```python
from build123d import *

# Parameters (mm, degrees)
SKETCH1_R           = 45
SKETCH1_R_2         = 1.2573
BOSS_EXTRUDE2_DEPTH = 2.5
BOSS_EXTRUDE4_START = -2.5
BOSS_EXTRUDE4_DEPTH = 2.5
CIRPATTERN1_COUNT   = 6
CUT_EXTRUDE2_DEPTH  = 2.5
SKETCH6_R           = 1.5
CUT_EXTRUDE3_DEPTH  = 5


with BuildPart() as part:
    # Sketch1 → Boss-Extrude2 (new body)
    with BuildSketch(Plane(origin=(0, 0, 0), x_dir=(1, 0, 0), z_dir=(0, 1, 0))):
        with Locations(Location((0, 0, 0), (0, 0, 270))):
            Circle(SKETCH1_R)
        with Locations(Location((-4.955, -33.87, 0), (0, 0, 270))):
            Circle(SKETCH1_R_2, mode=Mode.SUBTRACT)
        with Locations(Location((4.955, -33.87, 0), (0, 0, 90))):
            Circle(SKETCH1_R_2, mode=Mode.SUBTRACT)
        with Locations(Location((-4.955, 13.84, 0), (0, 0, 270))):
            Circle(SKETCH1_R_2, mode=Mode.SUBTRACT)
        with Locations(Location((4.955, 13.84, 0), (0, 0, 90))):
            Circle(SKETCH1_R_2, mode=Mode.SUBTRACT)
        Polygon((-9.9, -25), (-9.9, 0), (-9.9, 10), (9.9, 10), (9.9, 0), (9.9, -25), align=None, mode=Mode.SUBTRACT)
        with BuildLine():
            Line((-22.25, 22), (-22.25, -22))
            ThreePointArc((-22.25, -22), (-19.25, -25), (-16.25, -22))
            Line((-16.25, -22), (-16.25, 22))
            ThreePointArc((-16.25, 22), (-19.25, 25), (-22.25, 22))
        make_face(mode=Mode.SUBTRACT)
        with BuildLine():
            Line((16.25, 22), (16.25, -22))
            ThreePointArc((16.25, -22), (19.25, -25), (22.25, -22))
            Line((22.25, -22), (22.25, 22))
            ThreePointArc((22.25, 22), (19.25, 25), (16.25, 22))
        make_face(mode=Mode.SUBTRACT)
    extrude(amount=BOSS_EXTRUDE2_DEPTH)

    # Sketch2 → Boss-Extrude4 (add)
    with BuildSketch(Plane(origin=(0, 2.5, 0), x_dir=(1, 0, 0), z_dir=(0, 1, 0)).offset(BOSS_EXTRUDE4_START)):
        with BuildLine():
            ThreePointArc((-42.23454554, 15.532004475), (-45, 0), (-42.23454554, -15.532004475))
            add(Edge.make_bspline(
                [(-50.212380227, -7.942360629), (-45.3159648, -11.95963121), (-42.656686571, -14.489512492), (-42.23454554, -15.532004475)],
                knots=[0.089311832, 0.089311832, 0.089311832, 0.089311832, 1, 1, 1, 1], degree=3))
            ThreePointArc((-50.212380227, -7.942360629), (-54.5, 0), (-50.212380227, 7.942360629))
            add(Edge.make_bspline(
                [(-50.212380227, 7.942360629), (-45.3159648, 11.95963121), (-42.656686571, 14.489512492), (-42.23454554, 15.532004475)],
                knots=[0.089311832, 0.089311832, 0.089311832, 0.089311832, 1, 1, 1, 1], degree=3))
        make_face()
    boss_extrude4 = extrude(amount=BOSS_EXTRUDE4_DEPTH)

    # CirPattern1: Boss-Extrude4 ×6 about axis
    cirpattern1_axis = Axis((0, 2.5, 0), (0, 1, 0))
    for i in range(1, CIRPATTERN1_COUNT):
        add(boss_extrude4.rotate(cirpattern1_axis, i * 360 / CIRPATTERN1_COUNT))

    # Sketch5 → Cut-Extrude2 (cut)
    with BuildSketch(Plane(origin=(0, 2.5, 0), x_dir=(1, 0, 0), z_dir=(0, 1, 0))):
        with BuildLine():
            Line((-8.22468756, 44.342191593), (0, 46.65782144))
            Line((0, 46.65782144), (8.22468756, 44.342191593))
            ThreePointArc((8.22468756, 44.342191593), (0, 42.851652617), (-8.22468756, 44.342191593))
        make_face()
        with BuildLine():
            Line((40.406858652, 23.32891072), (42.513808159, 15.048307431))
            ThreePointArc((42.513808159, 15.048307431), (37.11061976, 21.425826308), (34.289120599, 29.293884161))
            Line((34.289120599, 29.293884161), (40.406858652, 23.32891072))
        make_face()
        with BuildLine():
            Line((40.406858652, -23.32891072), (34.289120599, -29.293884161))
            ThreePointArc((34.289120599, -29.293884161), (37.11061976, -21.425826308), (42.513808159, -15.048307431))
            Line((42.513808159, -15.048307431), (40.406858652, -23.32891072))
        make_face()
        with BuildLine():
            Line((0, -46.65782144), (-8.22468756, -44.342191593))
            ThreePointArc((-8.22468756, -44.342191593), (0, -42.851652617), (8.22468756, -44.342191593))
            Line((8.22468756, -44.342191593), (0, -46.65782144))
        make_face()
        with BuildLine():
            Line((-40.406858652, -23.32891072), (-42.513808159, -15.048307431))
            ThreePointArc((-42.513808159, -15.048307431), (-37.11061976, -21.425826308), (-34.289120599, -29.293884161))
            Line((-34.289120599, -29.293884161), (-40.406858652, -23.32891072))
        make_face()
        with BuildLine():
            Line((-40.406858652, 23.32891072), (-34.289120599, 29.293884161))
            ThreePointArc((-34.289120599, 29.293884161), (-37.11061976, 21.425826308), (-42.513808159, 15.048307431))
            Line((-42.513808159, 15.048307431), (-40.406858652, 23.32891072))
        make_face()
    extrude(amount=-CUT_EXTRUDE2_DEPTH, mode=Mode.SUBTRACT)

    # Sketch6 → Cut-Extrude3 (cut, symmetric)
    with BuildSketch(Plane(origin=(0, 2.5, 0), x_dir=(1, 0, 0), z_dir=(0, 1, 0))):
        with Locations(Location((-45, 0, 0), (0, 0, 270))):
            Circle(SKETCH6_R)
        with Locations(Location((-22.5, 38.97114317, 0), (0, 0, 270))):
            Circle(SKETCH6_R)
        with Locations(Location((22.5, 38.97114317, 0), (0, 0, 270))):
            Circle(SKETCH6_R)
        with Locations(Location((45, 0, 0), (0, 0, 270))):
            Circle(SKETCH6_R)
        with Locations(Location((22.5, -38.97114317, 0), (0, 0, 270))):
            Circle(SKETCH6_R)
        with Locations(Location((-22.5, -38.97114317, 0), (0, 0, 270))):
            Circle(SKETCH6_R)
    extrude(amount=CUT_EXTRUDE3_DEPTH, both=True, mode=Mode.SUBTRACT)


solid = part.part
```
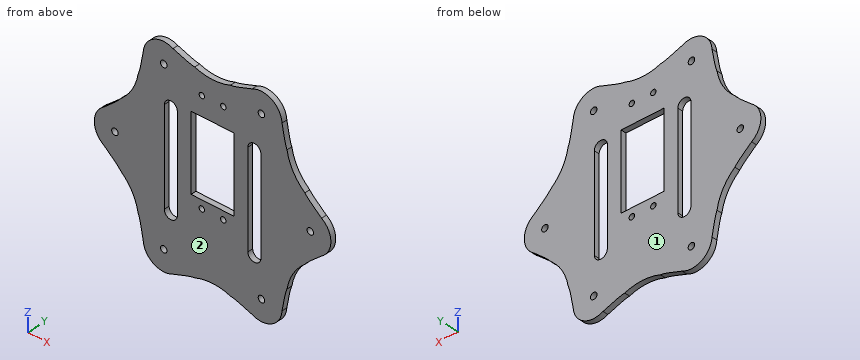
Source: CAD feature listing. Evaluate the final solid. Frame: model axes, mm. Face numbers are marked on the shaded views. Round coordinates to 2 decimals unless told otherwise and drop trailing zeros. Loops run counter-clockwise (first coordinate to the right, second up) from the corner with the lowest first, then second, coordinate; pieces in that order, holes last. Notation, with made-up numbers: M 58,-16.5 L 97,-16.5 A27 ccw 97,13.5 Z; hole C 85.5,-37.5 d7. An arc over 180 degrees is marked long. Use a Markdown table: item, result. Add a question column.
1. Section query B-B on z = 33.87. Give the number of separate pieces and of enclosed holes in the cut face, then the cut area to 3 significant figures.
2. Mould query, pull axis Y, two halves, no side actions, for the marked faces 1 and 2. Classes: pulls with the +Y half, pulls with the -Y half, needs draft (parallel to the pull), parting line crosses it, or undercut.
3. Section query A-A on x = 30.5. Return the cut outline in (y, z).
4. Contact query for flat-ended pins moving along their axis: P1, Ø1, axis at y = 1.5, z = 33.5, coming from the -X side; P2, Ø0.8, axis at y = 1.5, z = 10, coming from the -X side; P3, Ø0.8, axis at y = 1, z = -10.5, coming from the +X side. Output: stop coordinate, or through.
5. Line query: line 1 (X direction, y = 1.5, z = 0); line 2 (X direction, y = 2.15, z = -19); line 3 (X direction, y = 0.4, z = 18). Output: solid intervals per line, ascending.
Reported:
| question | item | result |
|---|---|---|
| 1 | separate pieces | 3 |
| 1 | enclosed holes | 0 |
| 1 | area | 153 mm² |
| 2 | face 1 | pulls with the +Y half |
| 2 | face 2 | pulls with the -Y half |
| 3 | outline | M 0,-44.09 L 2.5,-44.09 L 2.5,44.09 L 0,44.09 Z |
| 4 | P1 | stops at x = -33.21 |
| 4 | P2 | stops at x = -48.22 |
| 4 | P3 | stops at x = 47.63 |
| 5 | line 1 | x = -54.5 to -46.5, -43.5 to -22.25, -16.25 to -9.9, 9.9 to 16.25, 22.25 to 43.5, 46.5 to 54.5 |
| 5 | line 2 | x = -38.72 to -22.25, -16.25 to 16.25, 22.25 to 38.72 |
| 5 | line 3 | x = -39.52 to -22.25, -16.25 to -9.9, 9.9 to 16.25, 22.25 to 39.52 |
